Verification items for the finished model (mm, model axes). A direction names the side the tool comes from. Round coordinates to 2 decimals unless told otherwise and drop trailing zeros. Order: outer loops, then holes, each group sorted by start corner. A loop starts at its lowest first (then second) coordinate and runs counter-clockwise, first axis right, second up. Notation, with made-up numbers: (87.5, 31) -> (109.5, 31) arc R23 ccw to (109.5, 40) -> close; hole circle Ø11 at (82, 48). An arc over 180 degrees is marked (long way). Put each result on its own line as item: value.
from build123d import *

# Parameters (mm, degrees)
EXTRUDE_1_DEPTH           = 10
SKETCH_2_W                = 27
SKETCH_2_H                = 10
EXTRUDE_2_DEPTH           = 1.980559755
SKETCH_3_W                = 122.825116964
SKETCH_3_H                = 10
EXTRUDE_3_DEPTH           = 4
SKETCH_4_W                = 27
SKETCH_4_H                = 5
EXTRUDE_4_DEPTH           = 19
CUT_EXTRUDE_1_DEPTH       = 83.592386691
SKETCH_6_W                = 27
SKETCH_6_H                = 5
EXTRUDE_5_DEPTH           = 19
CUT_EXTRUDE_2_DEPTH       = 3
CUT_EXTRUDE_3_DEPTH       = 3
HOLE_WIZARD_4_0_4_1_D     = 4
HOLE_WIZARD_4_0_4_1_DEPTH = 44
HOLE_WIZARD_4_0_4_2_D     = 4


with BuildPart() as part:
    # Эскиз1 → Бобышка-Вытянуть1 (new body)
    with BuildSketch(Plane(origin=(0, 10, 0), x_dir=(1, 0, 0), z_dir=(0, 1, 0))):
        with BuildLine():
            Line((-13.5, -45.019440245), (13.5, -45.019440245))
            ThreePointArc((13.5, -45.019440245), (35.505543373, -30.795395594), (46.475800154, -7))
            Line((46.475800154, -7), (-46.475800154, -7))
            ThreePointArc((-46.475800154, -7), (-35.505543373, -30.795395594), (-13.5, -45.019440245))
        make_face()
    extrude(amount=-EXTRUDE_1_DEPTH)

    # Эскиз2 → Бобышка-Вытянуть2 (add)
    with BuildSketch(Plane.XY.offset(45.019440245)):
        with Locations((0, 5)):
            Rectangle(SKETCH_2_W, SKETCH_2_H)
    extrude(amount=EXTRUDE_2_DEPTH)

    # Эскиз3 → Бобышка-Вытянуть3 (add)
    with BuildSketch(Plane(origin=(0, 0, 7), x_dir=(-1, 0, 0), z_dir=(0, 0, -1))):
        with Locations((0, 5)):
            Rectangle(SKETCH_3_W, SKETCH_3_H)
    extrude(amount=EXTRUDE_3_DEPTH)

    # Эскиз4 → Бобышка-Вытянуть4 (add)
    with BuildSketch(Plane.XZ):
        with Locations((0, 44.5)):
            Rectangle(SKETCH_4_W, SKETCH_4_H)
    extrude(amount=EXTRUDE_4_DEPTH)

    # Эскиз5 → Вырез-Вытянуть1 (cut, through all)
    with BuildSketch(Plane(origin=(0, 10, 0), x_dir=(-1, 0, 0), z_dir=(0, 1, 0))):
        with BuildLine():
            Line((-41.412558482, 3), (41.412558482, 3))
            Line((41.412558482, 3), (41.412558482, 7))
            ThreePointArc((41.412558482, 7), (0, 42), (-41.412558482, 7))
            Line((-41.412558482, 7), (-41.412558482, 3))
        make_face()
    extrude(amount=-CUT_EXTRUDE_1_DEPTH, mode=Mode.SUBTRACT)

    # Эскиз6 → Бобышка-Вытянуть5 (add)
    with BuildSketch(Plane(origin=(0, 10, 0), x_dir=(-1, 0, 0), z_dir=(0, 1, 0))):
        with Locations((0, 44.5)):
            Rectangle(SKETCH_6_W, SKETCH_6_H)
    extrude(amount=EXTRUDE_5_DEPTH)

    # Эскиз7 → Вырез-Вытянуть2 (cut)
    with BuildSketch(Plane(origin=(0, 0, 42), x_dir=(-1, 0, 0), z_dir=(0, 0, -1))):
        Polygon((1.991858429, 26.95), (-1.991858429, 26.95), (-3.983716857, 23.5), (-1.991858429, 20.05), (1.991858429, 20.05), (3.983716857, 23.5), align=None)
    extrude(amount=-CUT_EXTRUDE_2_DEPTH, mode=Mode.SUBTRACT)

    # Эскиз8 → Вырез-Вытянуть3 (cut)
    with BuildSketch(Plane(origin=(0, 0, 42), x_dir=(-1, 0, 0), z_dir=(0, 0, -1))):
        Polygon((1.991858429, -10.05), (-1.991858429, -10.05), (-3.983716857, -13.5), (-1.991858429, -16.95), (1.991858429, -16.95), (3.983716857, -13.5), align=None)
    extrude(amount=-CUT_EXTRUDE_3_DEPTH, mode=Mode.SUBTRACT)

    # Диаметр отверстия Ø4.0 (4)1
    with Locations(Plane.XY.offset(47)):
        with Locations((0, 23.5), (0, -13.5)):
            Hole(HOLE_WIZARD_4_0_4_1_D / 2, depth=HOLE_WIZARD_4_0_4_1_DEPTH)

    # Диаметр отверстия Ø4.0 (4)2 (through all)
    with Locations(Plane.XY.offset(7)):
        with Locations((-54.412558482, 5), (54.412558482, 5)):
            Hole(HOLE_WIZARD_4_0_4_2_D / 2)


solid = part.part
Item 1: Release check for a two-part mould opening along X. For faces 1 (the flat face through (-61.413, 5, 5)), 2 (the flat face through (3, 21.8, 43.5)), 3 (the flat face through (3, 25.2, 43.5)), 4 (the flat face through (0, 5, 47)) record: +X half, -X half, draft (parallel to the pull), parting line (faces both ways), or undercut.
Check sheet entries:
face 1: -X half
face 2: undercut
face 3: undercut
face 4: draft
Item 2: Gauge pin test, flat ends, axial feed: pin 1 Ø3 at (x, y) = (-53.5, 4.5) entering from +Z; pin 2 Ø5.5 at (x, y) = (-1.5, -12.5) entering from -Z; pin 3 Ø6 at (x, z) = (47, 16) entering from -Y; pin 4 Ø5 at (x, z) = (10, 40.5) entering from +Y. Record the tip position at first contact, or that the pin passes through.
Check sheet entries:
pin 1: stops at z = 7
pin 2: stops at z = 42
pin 3: stops at y = 0
pin 4: stops at y = 29
Item 3: Material ranges on L1, parallel to Y at x = 0, z = 45.6; L2, parallel to Z at x = -7, y = 15; L3, parallel to Y at x = -51, z = 6.5, recorded low to high. Write a range as [from, to].
Check sheet entries:
L1: y = [-19, -15.5], [-11.5, 21.5], [25.5, 29]
L2: z = [42, 47]
L3: y = [0, 10]
Item 4: Section check D-D on x = -39. Record the boundary of the cut face in (y, z), then the cut area to 3 significant figures.
Check sheet entries:
outline: (0, 15.59) -> (10, 15.59) -> (10, 26.23) -> (0, 26.23) -> close
area: 106 mm^2
Item 5: Section check B-B on z = 18.5. Record the boundary of the cut face in (x, y).
Check sheet entries:
outline: (-43.21, 0) -> (-37.71, 0) -> (-37.71, 10) -> (-43.21, 10) -> close; (37.71, 0) -> (43.21, 0) -> (43.21, 10) -> (37.71, 10) -> close
Item 6: Section check C-C on x = 37.5. Record the boundary of the cut face in (y, z).
Check sheet entries:
outline: (0, 18.91) -> (10, 18.91) -> (10, 28.33) -> (0, 28.33) -> close
Item 7: Tool access check on faces 5 (the flat face through (-3, 21.8, 43.5)), 6 (the flat face through (52, 5, 7)), 7 (the cylindrical face through (-0.923, 21.726, 45.986)), 8 (the flat face through (0, -9, 42)), 9 (the flat face through (41.413, 5, 5)). Record the directions out of +Z, -Z, +X, -X, +Y, -Y that give a thin tool (end or side, any length) a straight path to the whole face; none if there is none.
Check sheet entries:
face 5: -Z
face 6: +Z, +X, +Y, -Y
face 7: +Z, -Z
face 8: -Z, +X, -X, -Y
face 9: -Z, +Y, -Y
Item 8: Section check A-A on z = 29. Record the boundary of the cut face in (x, y).
Check sheet entries:
outline: (-36.99, 0) -> (-30.38, 0) -> (-30.38, 10) -> (-36.99, 10) -> close; (30.38, 0) -> (36.99, 0) -> (36.99, 10) -> (30.38, 10) -> close
